For this review, use the dimensioned drawing (mm, ordinates from the lowest corner) and the shaded views. Coordinates: 2 decimals unless noted, no trailing zeros. Order: outer loops, then holes, each group sorted by start corner. A loop starts at its lowest first (then second) coordinate and runs counter-clockwise, first axis right, second up. Notation, with made-up numbers: M -33,20 L 8,20 A18 ccw 8,31 Z; hole C -15.5,27 d1. An arc over 180 degrees is marked long. Use one line per item in the form item = value. Start each with the question number.
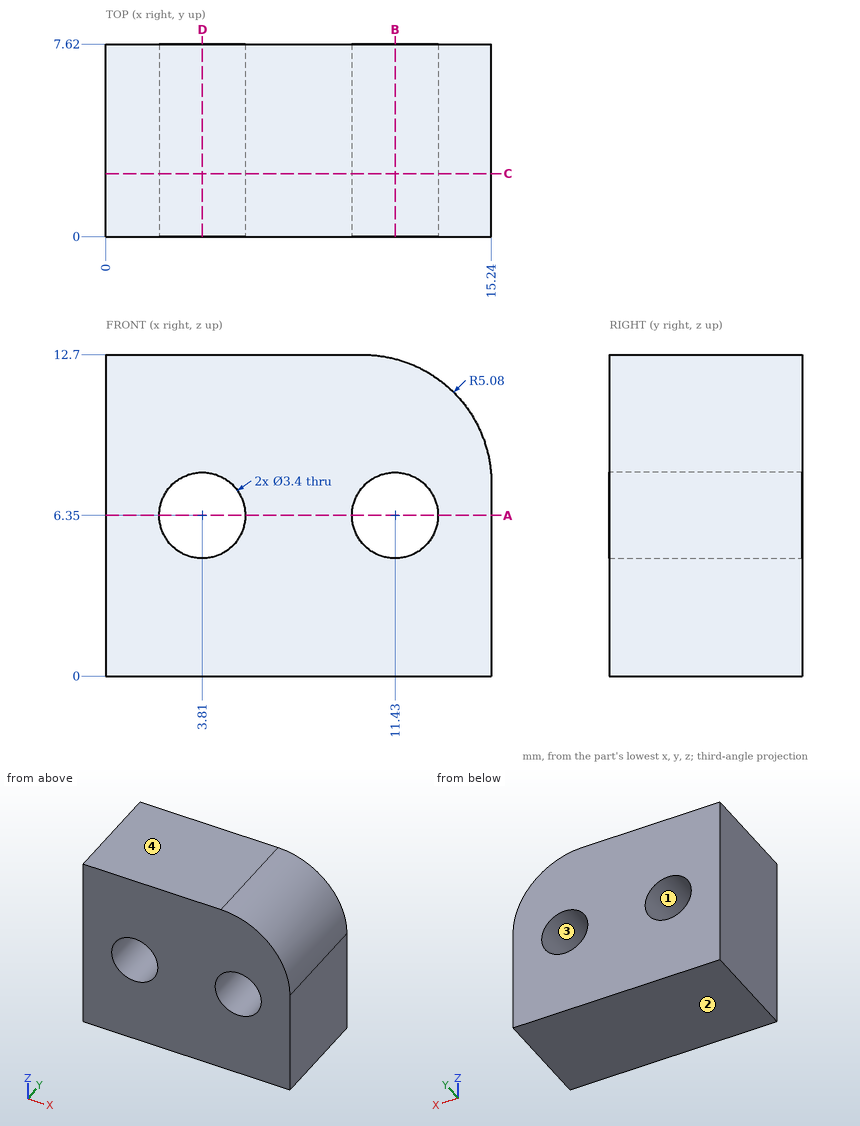
1. Consider section B-B, the plane x = 11.43. Write out the cut boundary in (y, z).
2. Consider section C-C, the plane y = 2.5. Write out the cut boundary in (x, z).
3. Consider section D-D, the plane x = 3.81. Write out the cut boundary in (y, z).
4. Consider section A-A, the plane z = 6.35. Write out the cut boundary in (x, y), plus the area to 3 significant figures.
5. The part is to be moulded in two halves that separate along Z. For the marked faces 1, 2, 3 and 4, say which applies: pulls with the +Z half, pulls with the -Z half, needs draft (parallel to the pull), parting line crosses it, or undercut.
6. For pin 1 Ø3 at (x, z) = (11.43, 6.35) entering from -Y, flat-tipped, find the tip position at first contact; note if it passes through.
7. To check wall thickness, follow line 1 (X direction, y = 5, z = 6.35); line 2 (Z direction, x = 5, y = 3.25); line 3 (Z direction, x = 11.43, y = 2.5). State the ranges of each line that lie inside material, in increasing order.
Answers follow:
q1.outline = M 0,0 L 7.62,0 L 7.62,4.65 L 0,4.65 Z; M 0,8.05 L 7.62,8.05 L 7.62,12.54 L 0,12.54 Z
q2.outline = M 0,0 L 15.24,0 L 15.24,7.62 A5.08 ccw 10.16,12.7 L 0,12.7 Z; hole C 3.81,6.35 d3.4; hole C 11.43,6.35 d3.4
q3.outline = M 0,0 L 7.62,0 L 7.62,4.65 L 0,4.65 Z; M 0,8.05 L 7.62,8.05 L 7.62,12.7 L 0,12.7 Z
q4.outline = M 0,0 L 2.11,0 L 2.11,7.62 L 0,7.62 Z; M 5.51,0 L 9.73,0 L 9.73,7.62 L 5.51,7.62 Z; M 13.13,0 L 15.24,0 L 15.24,7.62 L 13.13,7.62 Z
q4.area = 64.3 mm²
q5.face_1 = undercut
q5.face_2 = pulls with the -Z half
q5.face_3 = undercut
q5.face_4 = pulls with the +Z half
q6.pin_1 = through
q7.line_1 = 0 to 2.11, 5.51 to 9.73, 13.13 to 15.24
q7.line_2 = 0 to 5.14, 7.56 to 12.7
q7.line_3 = 0 to 4.65, 8.05 to 12.54
